The listing builds one solid part. Answer for the finished solid, in the listing's coordinates (mm). A direction names the side the tool comes from. Round coordinates to 2 decimals unless told otherwise and drop trailing zeros. Write each loop counter-clockwise with the first axis right and the second up, starting at its lowest first coordinate (ties: lowest second). Pieces come first, ordered by that corner, then holes.
from build123d import *

# Parameters (mm, degrees)
SKETCH1_R             = 11.938
BOSS_EXTRUDE1_DEPTH   = 19.05
SKETCH2_R             = 1.177518958
BOSS_EXTRUDE2_DEPTH   = 0.304204724
SKETCH2_R_2           = 1.16518976
BOSS_EXTRUDE2_2_DEPTH = 0.304204724
SKETCH3_W             = 28.109952108
SKETCH3_H             = 2.33037952
BOSS_EXTRUDE3_DEPTH   = 0.254
SKETCH4_R             = 0.795236377
CUT_EXTRUDE1_DEPTH    = 0.905720074
SKETCH5_R             = 0.753950063
CUT_EXTRUDE2_DEPTH    = 1.016
SKETCH6_R             = 0.47077468
BOSS_EXTRUDE4_DEPTH   = 0.245031324
SKETCH8_R             = 3.743161578
BOSS_EXTRUDE5_DEPTH   = 3.302


with BuildPart() as part:
    # Sketch1 → Boss-Extrude1 (new body)
    with BuildSketch(Plane.XY):
        Circle(SKETCH1_R)
    extrude(amount=BOSS_EXTRUDE1_DEPTH)



with BuildPart() as body_2:
    # Sketch2 → Boss-Extrude2 (new body)
    with BuildSketch(Plane(origin=(0, 0, 0), x_dir=(-1, 0, 0), z_dir=(0, 0, -1))):
        with Locations((13.97, 0)):
            Circle(SKETCH2_R)
    extrude(amount=-BOSS_EXTRUDE2_DEPTH)


with BuildPart() as body_3:
    # Sketch2 → Boss-Extrude2 2 (new body)
    with BuildSketch(Plane(origin=(0, 0, 0), x_dir=(-1, 0, 0), z_dir=(0, 0, -1))):
        with Locations((-13.97, 0)):
            Circle(SKETCH2_R_2)
    extrude(amount=-BOSS_EXTRUDE2_2_DEPTH)


with BuildPart() as part_1:
    add(part.part)

    add(body_2.part)  # Boss-Extrude3 merges body 2

    add(body_3.part)  # Boss-Extrude3 merges body 3
    # Sketch3 → Boss-Extrude3 (add)
    with BuildSketch(Plane(origin=(0, 0, 0), x_dir=(-1, 0, 0), z_dir=(0, 0, -1))):
        with Locations((0.084976054, 0)):
            Rectangle(SKETCH3_W, SKETCH3_H)
    extrude(amount=-BOSS_EXTRUDE3_DEPTH)

    # Sketch4 → Cut-Extrude1 (cut)
    with BuildSketch(Plane(origin=(0, 0, 0), x_dir=(-1, 0, 0), z_dir=(0, 0, -1))):
        with Locations((-13.97, 0)):
            Circle(SKETCH4_R)
    extrude(amount=-CUT_EXTRUDE1_DEPTH, mode=Mode.SUBTRACT)

    # Sketch5 → Cut-Extrude2 (cut)
    with BuildSketch(Plane(origin=(0, 0, 0), x_dir=(-1, 0, 0), z_dir=(0, 0, -1))):
        with Locations((13.97, 0)):
            Circle(SKETCH5_R)
    extrude(amount=-CUT_EXTRUDE2_DEPTH, mode=Mode.SUBTRACT)

    # Sketch6 → Boss-Extrude4 (add)
    with BuildSketch(Plane(origin=(0, 0, 0), x_dir=(-1, 0, 0), z_dir=(0, 0, -1))):
        with Locations((0, 6.604)):
            Circle(SKETCH6_R)
    extrude(amount=BOSS_EXTRUDE4_DEPTH)

    # Sketch8 → Boss-Extrude5 (add)
    with BuildSketch(Plane(origin=(0, 0, -0.245031324), x_dir=(-1, 0, 0), z_dir=(0, 0, -1))):
        with Locations((0, 6.604)):
            Circle(SKETCH8_R)
    extrude(amount=BOSS_EXTRUDE5_DEPTH)


solid = part_1.part
1. Section C-C on z = 2.25 is taken. Determine the outline of the cut face in (x, y).
Geometry says:
outline: circle Ø23.88 at (0, 0)
2. Straight lines are drawn through the part: line 1 along Y through (x, z) = (-13.97, 0.1); line 2 along Z through (x, y) = (3, 5.25); line 3 along Z through (x, y) = (-1.5, -0.25). For each, find the intervals that lie inside material, in ascending order.
Geometry says:
line 1: y = -1.18 to -0.75, 0.75 to 1.18
line 2: z = -3.55 to -0.25, 0 to 19.05
line 3: z = 0 to 19.05
3. Section B-B on x = -3 is taken. Determine the outline of the cut face in (y, z).
Geometry says:
outline: (-11.55, 0) - (11.55, 0) - (11.55, 19.05) - (-11.55, 19.05) - close; (4.37, -3.55) - (8.84, -3.55) - (8.84, -0.25) - (4.37, -0.25) - close
4. Section A-A on y = 0 is taken. Determine the outline of the cut face in (x, z).
Geometry says:
outline: (-15.15, 0) - (-14.72, 0) - (-14.72, 0.3) - (-15.15, 0.3) - close; (-13.22, 0) - (13.17, 0) - (13.17, 0.3) - (12.8, 0.3) - (12.8, 0.25) - (11.94, 0.25) - (11.94, 19.05) - (-11.94, 19.05) - (-11.94, 0.25) - (-12.79, 0.25) - (-12.79, 0.3) - (-13.22, 0.3) - close; (14.77, 0) - (15.14, 0) - (15.14, 0.3) - (14.77, 0.3) - close
5. For a pull along X with two mould halves and no side action, classify faces 1 (the face through (12.5, 0, 0.254)), 2 (the face through (14, -1, 0.304)), 3 (the face through (-13.217, 0.033, 0.15)), 4 (the face through (0.487, 10.315, -1.873)) as released by +X, released by -X, zero draft, split by the parting line, or undercut.
Geometry says:
face 1: undercut
face 2: zero draft
face 3: undercut
face 4: split by the parting line
6. A tool of negligible diameter and unlimited length cuts with its end or side. For faces 5 (the face through (-12.4, 0, 0.254)), 6 (the face through (-14, -1, 0.304)), 7 (the face through (0, 0, 19.05)), from which of +Z, -Z, +X, -X, +Y, -Y can it reach the whole face along a straight path? Write none if from no direction.
Geometry says:
face 5: +Z
face 6: +Z, -X, +Y, -Y
face 7: +Z, +X, -X, +Y, -Y
7. Given pin 1 (12 mm diameter, centred on y = 8.5, z = 15.5, fed in from -X); pin 2 (4 mm diameter, centred on x = 11.5, y = 6.5, fed in from -Z); pin 3 (3 mm diameter, centred on y = 8.5, z = 4.5, fed in from -X); pin 4 (1.2 mm diameter, centred on x = -13.97, y = 0, fed in from -Z), each flat-ended and moving along its own axis, determine where each tip first touches the part or whether it passes through.
Geometry says:
pin 1: stops at x = -11.67
pin 2: stops at z = 0
pin 3: stops at x = -9.67
pin 4: passes through
8. Section D-D on x = 2 is taken. Determine the outline of the cut face in (y, z), plus the area to 3 significant figures.
Geometry says:
outline: (-11.77, 0) - (11.77, 0) - (11.77, 19.05) - (-11.77, 19.05) - close; (3.44, -3.55) - (9.77, -3.55) - (9.77, -0.25) - (3.44, -0.25) - close
area: 469 mm2
